Here's how the part is built. I have some questions about the finished solid (model axes, mm). Face numbers are marked on the shaded views. A direction names the side the tool comes from. Coordinates: 2 decimals unless noted, no trailing zeros. Order: outer loops, then holes, each group sorted by start corner. A loop starts at its lowest first (then second) coordinate and runs counter-clockwise, first axis right, second up. Notation, with made-up numbers: (-21.5, -8) - (24.5, -8) arc R13 cw to (24.5, -4) - close; hole circle Ø6 at (78, 43). An arc over 180 degrees is marked (long way). Answer as CSV lines item,"result". Start each with the question number.
Q1. Suppose I cut it at A-A (z = 0). Please give me the cut outline in (x, y).
Q2. Suppose I cut it at C-C (x = 0). Please give me the cut outline in (y, z), then the cut area to 3 significant figures.
Q3. Thinking about a two-plate mould opening in Z: for the marked faces 1, 2, 3 and 4, which applies, released by +Z, released by -Z, zero draft, split by the parting line, or undercut?
Q4. Suppose I cut it at D-D (y = -208). Please give me the cut outline in (x, z).
Q5. I need wall thicknesses on line 1 (Y direction, x = 0, z = 59); line 2 (Z direction, x = 75, y = -182.5); line 3 (Z direction, x = 18, y = -106). Which ranges of each line are inside material? Lowest first, please.
Q6. For the marked faces 5 and 6, which set-ups out of +Z, -Z, +X, -X, +Y, -Y let a thin tool reach every point of the face, with its end or its side?
Q7. Suppose I cut it at B-B (y = -162.5). Please give me the cut outline in (x, z), then the cut area to 3 significant figures.
Q8. For pin 1 Ø6 at (x, z) = (-59.5, -29.5) entering from +Y; pin 2 Ø2 at (x, z) = (49, 59) entering from +Y; pin 3 Ø8 at (x, z) = (-58.5, -37.5) entering from +Y, each with a flat end and sliding along its axis, tell me the tip position at first contact or that it passes through.
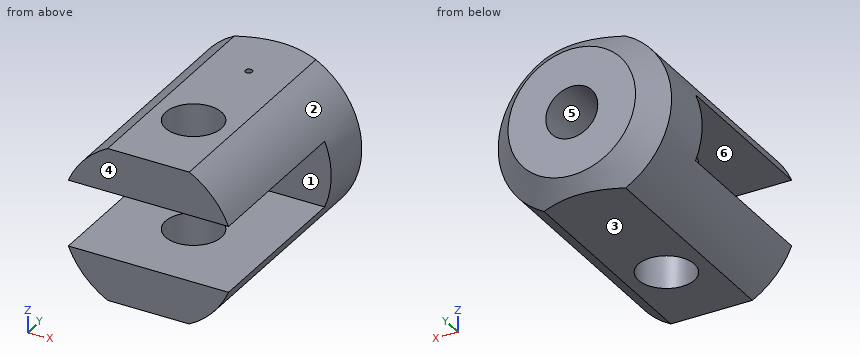
from build123d import *

# Parameters (mm, degrees)
SKETCH_1_R          = 85
EXTRUDE_1_DEPTH     = 240
SKETCH_2_W          = 162
SKETCH_2_H          = 14
CUT_EXTRUDE_1_DEPTH = 269.421310629
SKETCH_5_W          = 188
SKETCH_5_H          = 65
CUT_EXTRUDE_2_DEPTH = 165
SKETCH_6_R          = 27.5
CUT_EXTRUDE_3_DEPTH = 296.508037116
SKETCH_6_3_R        = 3.4
CUT_EXTRUDE_4_DEPTH = 20
CUT_EXTRUDE_5_REACH = 267.424
SKETCH_8_R          = 25.5


with BuildPart() as part:
    # Sketch 1 → Extrude 1 (new body)
    with BuildSketch(Plane(origin=(0, 0, 0), x_dir=(1, 0, 0), z_dir=(0, 1, 0))):
        with Locations(Location((0, 0, 0), (0, 0, 270))):
            Circle(SKETCH_1_R)
    extrude(amount=-EXTRUDE_1_DEPTH)

    # Sketch 2 → Cut-Extrude 1 (cut, through all)
    with BuildSketch(Plane(origin=(0, 0, 0), x_dir=(1, 0, 0), z_dir=(0, 1, 0))):
        with Locations((1.586849721, 82)):
            Rectangle(SKETCH_2_W, SKETCH_2_H)
    cut_extrude_1 = extrude(amount=-CUT_EXTRUDE_1_DEPTH, mode=Mode.SUBTRACT)

    # Mirror 1: Cut-Extrude 1 across plane
    add(cut_extrude_1.mirror(Plane.XY), mode=Mode.SUBTRACT)

    # Sketch 3 → Cut-Revolve 1 (revolve, cut)
    with BuildSketch(Plane.XY, mode=Mode.PRIVATE) as cut_revolve_1_sk:
        Polygon((85, -22.5), (62.5, 0), (85, 0), align=None)
    revolve(cut_revolve_1_sk.sketch.rotate(Axis((0, -240, 0), (0, 1, 0)), 90), axis=Axis((0, -240, 0), (0, 1, 0)), mode=Mode.SUBTRACT)

    # Sketch 5 → Cut-Extrude 2 (cut)
    with BuildSketch(Plane.XZ.offset(240)):
        Rectangle(SKETCH_5_W, SKETCH_5_H)
    extrude(amount=-CUT_EXTRUDE_2_DEPTH, mode=Mode.SUBTRACT)

    # Sketch 6 → Cut-Extrude 3 (cut, through all)
    with BuildSketch(Plane.XY.offset(75)):
        with Locations((0, -162.5)):
            Circle(SKETCH_6_R)
    extrude(amount=-CUT_EXTRUDE_3_DEPTH, mode=Mode.SUBTRACT)

    # Sketch 6_3 → Cut-Extrude 4 (cut)
    with BuildSketch(Plane.XY.offset(75)):
        with Locations((0, -67.5)):
            Circle(SKETCH_6_3_R)
    extrude(amount=-CUT_EXTRUDE_4_DEPTH, mode=Mode.SUBTRACT)

    # Sketch 8 → Cut-Extrude 5 (cut, up to next)
    with BuildSketch(Plane(origin=(0, 0, 0), x_dir=(1, 0, 0), z_dir=(0, 1, 0)), mode=Mode.PRIVATE) as cut_extrude_5_sk1:
        with Locations(Location((0, 0, 0), (0, 0, 270))):
            Circle(SKETCH_8_R)
    cut_extrude_5_tool1 = extrude(cut_extrude_5_sk1.sketch, amount=-CUT_EXTRUDE_5_REACH, mode=Mode.PRIVATE) & part.part
    add(cut_extrude_5_tool1.solids().sort_by_distance((0, 0, 0))[0], mode=Mode.SUBTRACT)


solid = part.part
Here are the results:
1,outline,"(-85, -75) - (-25.5, -75) - (-25.5, 0) - (-62.5, 0) - (-85, -22.5) - close; (25.5, -75) - (85, -75) - (85, -22.5) - (62.5, 0) - (25.5, 0) - close"
2,outline,"(-240, -75) - (-190, -75) - (-190, -32.5) - (-240, -32.5) - close; (-240, 32.5) - (-190, 32.5) - (-190, 75) - (-240, 75) - close; (-135, -75) - (-12.5, -75) - (0, -62.5) - (0, -25.5) - (-75, -25.5) - (-75, -32.5) - (-135, -32.5) - close; (-135, 32.5) - (-75, 32.5) - (-75, 25.5) - (0, 25.5) - (0, 62.5) - (-12.5, 75) - (-64.1, 75) - (-64.1, 55) - (-70.9, 55) - (-70.9, 75) - (-135, 75) - close"
2,area,"16,500 mm²"
3,face 1,"undercut"
3,face 2,"split by the parting line"
3,face 3,"released by -Z"
3,face 4,"zero draft"
4,outline,"(-78.54, -32.5) arc R85 ccw to (-40, -75) - (40, -75) arc R85 ccw to (78.54, -32.5) - close; (-78.54, 32.5) - (78.54, 32.5) arc R85 ccw to (40, 75) - (-40, 75) arc R85 ccw to start"
5,line 1,"y = -240 to -190, -135 to -70.9, -64.1 to 0"
5,line 2,"z = -40 to -32.5, 32.5 to 40"
5,line 3,"z = -75 to -32.5, 32.5 to 75"
6,face 5,"+Y, -Y"
6,face 6,"+X, -X, -Y"
7,outline,"(-78.54, -32.5) arc R85 ccw to (-40, -75) - (-27.5, -75) - (-27.5, -32.5) - close; (-78.54, 32.5) - (-27.5, 32.5) - (-27.5, 75) - (-40, 75) arc R85 ccw to start; (27.5, -75) - (40, -75) arc R85 ccw to (78.54, -32.5) - (27.5, -32.5) - close; (27.5, 32.5) - (78.54, 32.5) arc R85 ccw to (40, 75) - (27.5, 75) - close"
7,area,"6,170 mm²"
8,pin 1,"stops at y = -0.91"
8,pin 2,"stops at y = -13.19"
8,pin 3,"stops at y = -2.99"
